Design review of the part shown in the three views and the two pictorial views. Dimensions are in mm from the part's minimum x, y and z. A direction names the side the tool comes from. Give positions to 0.01 mm unless a question says otherwise; leave off trailing zeros. Loops run counter-clockwise (first coordinate to the right, second up) from the corner with the lowest first, then second, coordinate; pieces in that order, holes last. Notation, with made-up numbers: M 66,-38.5 L 120,-38.5 A22 ccw 120,-7.5 Z; hole C 61,-8 d3. An arc over 180 degrees is marked long. Return JSON: item names as keys, results as strings. Group by question number.
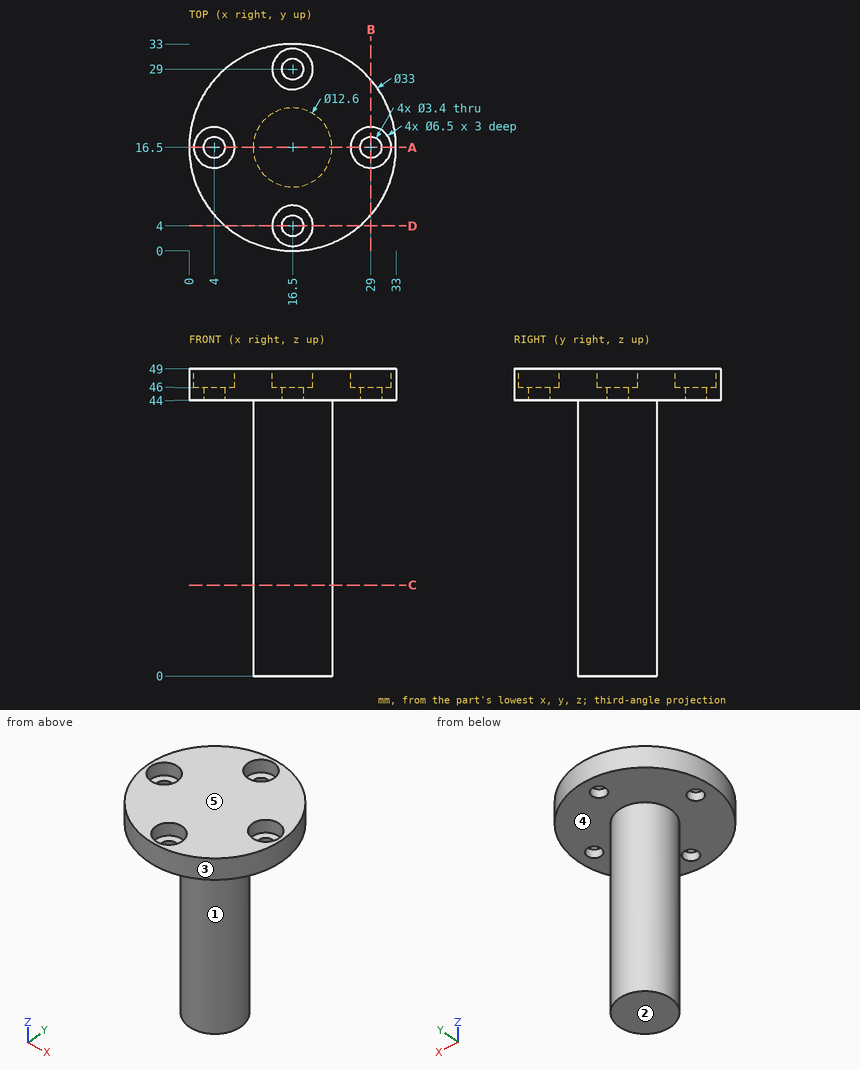
(1) Mouldability with a two-part tool opening along Z and no side actions: class the marked faces 3, 4 and 5 as released by +Z, released by -Z, zero draft, split by the parting line, or undercut.
(2) Add section A-A (y = 16.5). Write out the cut boundary in (x, z), and give its area (3 significant figures).
(3) Add section B-B (x = 29). Write out the cut boundary in (y, z).
(4) Add section C-C (z = 14.5). Write out the cut boundary in (x, y), and give its area (3 significant figures).
(5) For probe 1 along Z at (x, y) = (23.5, 28); probe 2 along Y at (x, z) = (4, 45.55); probe 3 along Y at (x, z) = (16, 47), list the stretches that pass through material, from the lowest coordinate up.
(6) For the marked faces 1 and 2, list the 3-axis set-ups (+Z, -Z, +X, -X, +Y, -Y) from which the entire face can be reached by the end or side of a thin tool; tool diameter is ignored.
(7) For pin 1 (12 mm diameter, centred on x = 16.5, y = 3.5, fed in from -Z); pin 2 (1 mm diameter, centred on x = 22, z = 25.5, fed in from -Y); pin 3 (2 mm diameter, centred on x = 30, y = 15, fed in from +Z), all flat-tipped, find the tip position at first contact; note any pin that passes through.
Verdict:
{
 "1": {"face 3": "zero draft", "face 4": "released by -Z", "face 5": "released by +Z"},
 "2": {"outline": "M 0,44 L 2.3,44 L 2.3,46 L 0.75,46 L 0.75,49 L 0,49 Z; M 5.7,44 L 10.2,44 L 10.2,0 L 22.8,0 L 22.8,44 L 27.3,44 L 27.3,46 L 25.75,46 L 25.75,49 L 7.25,49 L 7.25,46 L 5.7,46 Z; M 30.7,44 L 33,44 L 33,49 L 32.25,49 L 32.25,46 L 30.7,46 Z", "area": "667 mm²"},
 "3": {"outline": "M 5.73,44 L 14.8,44 L 14.8,46 L 13.25,46 L 13.25,49 L 5.73,49 Z; M 18.2,44 L 27.27,44 L 27.27,49 L 19.75,49 L 19.75,46 L 18.2,46 Z"},
 "4": {"outline": "C 16.5,16.5 d12.6", "area": "125 mm²"},
 "5": {"probe 1": "z = 44 to 49", "probe 2": "y = 5.73 to 14.8, 18.2 to 27.27", "probe 3": "y = 0.01 to 0.79, 7.21 to 25.79, 32.21 to 32.99"},
 "6": {"face 1": "-Z", "face 2": "-Z, +X, -X, +Y, -Y"},
 "7": {"pin 1": "stops at z = 44", "pin 2": "stops at y = 12.67", "pin 3": "stops at z = 46"}
}
